Work out the finished part from the listing and answer in its coordinate system (mm). Face numbers are marked on the shaded views. A direction names the side the tool comes from. Round coordinates to 2 decimals unless told otherwise and drop trailing zeros. Order: outer loops, then holes, each group sorted by start corner. A loop starts at its lowest first (then second) coordinate and runs counter-clockwise, first axis right, second up. Notation, with made-up numbers: (71.5, -37) -> (105.5, -37) arc R23 ccw to (105.5, -10) -> close; hole circle Ø8 at (56.5, 5). An arc over 180 degrees is marked (long way). Use a Markdown table: item, result. Add a question column.
Item 1: A tool of negligible diameter and unlimited length cuts with its end or side. For the marked faces 1, 2 and 3, from which of +Z, -Z, +X, -X, +Y, -Y can it reach the whole face along a straight path? Write none if from no direction.
Item 2: A cutting plane is placed at A-A, the plane x = 5.85. Determine the outline of the cut face in (y, z).
Item 3: A cutting plane is placed at D-D, the plane z = 13. Determine the outline of the cut face in (x, y).
Item 4: Flat-ended cylindrical pins translate along their axes: P1, Ø5.5, axis at x = 7, z = 21, coming from the +Y side; P2, Ø2, axis at y = 5, z = 11, coming from the +X side; P3, Ø0.8, axis at x = 6, y = 8.5, coming from the +Z side. Find the tip coordinate at first contact, or state that the pin passes through.
Item 5: A cutting plane is placed at B-B, the plane y = 6. Determine the outline of the cut face in (x, z).
Item 6: Find the intervals of material crossed by L1, parallel to Z at x = 10, y = 5; L2, parallel to X at y = 6, z = 20.75; L3, parallel to X at y = 4.5, z = 14.5, in increasing order. Write a range as [from, to].
Item 7: A cutting plane is placed at C-C, the plane z = 5.5. Determine the outline of the cut face in (x, y), plus the area to 3 significant figures.
from build123d import *

# Parameters (mm, degrees)
SKETCH_1_W          = 11.7
SKETCH_1_H          = 12
EXTRUDE_1_DEPTH     = 4.5
SKETCH_2_R          = 3.5
EXTRUDE_2_DEPTH     = 7
SKETCH_3_R          = 3
EXTRUDE_3_DEPTH     = 13
CUT_EXTRUDE_START   = -10
CUT_EXTRUDE_1_DEPTH = 10
FILLET_1_R          = 0.5


with BuildPart() as part:
    # 草图1 → 凸台-拉伸1 (new body)
    with BuildSketch(Plane.XY):
        with Locations((5.85, 6)):
            Rectangle(SKETCH_1_W, SKETCH_1_H)
    extrude(amount=EXTRUDE_1_DEPTH)

    # 草图2 → 凸台-拉伸2 (add)
    with BuildSketch(Plane.XY.offset(4.5)):
        with Locations((5.85, 6)):
            Circle(SKETCH_2_R)
    extrude(amount=EXTRUDE_2_DEPTH)

    # 草图3 → 凸台-拉伸3 (add)
    with BuildSketch(Plane.XY.offset(11.5)):
        with Locations(Location((5.85, 6, 0), (0, 0, 180))):
            Circle(SKETCH_3_R)
    extrude(amount=EXTRUDE_3_DEPTH)

    # 草图4 → 切除-拉伸1 (cut)
    with BuildSketch(Plane.XY.offset(24.5).offset(CUT_EXTRUDE_START)):
        with BuildLine():
            Line((3.251923789, 7.5), (8.448076211, 7.5))
            ThreePointArc((8.448076211, 7.5), (5.85, 9), (3.251923789, 7.5))
        make_face()
    extrude(amount=CUT_EXTRUDE_1_DEPTH, mode=Mode.SUBTRACT)

    # 圆角1
    fillet_1_edges = [part.edges().sort_by_distance(p)[0] for p in [
        (2.35, 6, 4.5),
    ]]
    fillet(fillet_1_edges, radius=FILLET_1_R)


solid = part.part
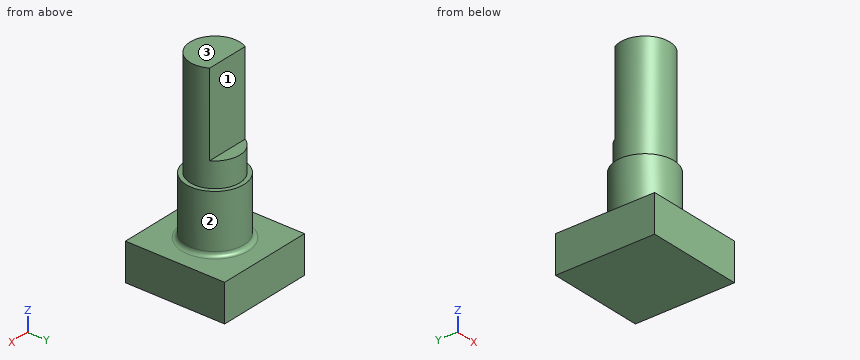
Reported:
| question | item | result |
|---|---|---|
| 1 | face 1 | +Z, +X, -X, +Y |
| 1 | face 2 | +Z |
| 1 | face 3 | +Z, +X, -X, +Y, -Y |
| 2 | outline | (0, 0) -> (12, 0) -> (12, 4.5) -> (10, 4.5) arc R0.5 cw to (9.5, 5) -> (9.5, 11.5) -> (9, 11.5) -> (9, 14.5) -> (7.5, 14.5) -> (7.5, 24.5) -> (3, 24.5) -> (3, 11.5) -> (2.5, 11.5) -> (2.5, 5) arc R0.5 cw to (2, 4.5) -> (0, 4.5) -> close |
| 3 | outline | circle Ø6 at (5.85, 6) |
| 4 | P1 | y = 7.5 |
| 4 | P2 | x = 9.35 |
| 4 | P3 | z = 14.5 |
| 5 | outline | (0, 0) -> (11.7, 0) -> (11.7, 4.5) -> (9.85, 4.5) arc R0.5 cw to (9.35, 5) -> (9.35, 11.5) -> (8.85, 11.5) -> (8.85, 24.5) -> (2.85, 24.5) -> (2.85, 11.5) -> (2.35, 11.5) -> (2.35, 5) arc R0.5 cw to (1.85, 4.5) -> (0, 4.5) -> close |
| 6 | L1 | [0, 4.5] |
| 6 | L2 | [2.85, 8.85] |
| 6 | L3 | [3.25, 8.45] |
| 7 | outline | circle Ø7 at (5.85, 6) |
| 7 | area | 38.5 mm² |
